Here's how the part is built. I have some questions about the finished solid (model axes, mm). A direction names the side the tool comes from. Coordinates: 2 decimals unless noted, no trailing zeros. Order: outer loops, then holes, each group sorted by start corner. A loop starts at its lowest first (then second) coordinate and runs counter-clockwise, first axis right, second up. Notation, with made-up numbers: (23.25, 82) - (77.25, 82) arc R32 ccw to (77.25, 108) - close; hole circle Ø7 at (81.25, -1). An arc over 180 degrees is marked (long way). Answer as CSV lines item,"result". Start each with the question number.
Item 1: We'd pull the mould along X, two halves only. Please class faces 4 (the face through (17.092, 32, 5)), 5 (the face through (16.52, 59.32, 1.97)), 6 (the face through (19.435, 52, 2)): pulls with the +X half, pulls with the -X half, needs draft (parallel to the pull), parting line crosses it, or undercut.
Item 2: Imagine slicing it at A-A on z = 8. List the corners of the cut face in (x, y) for me, and give its area (3 significant figures).
Item 3: Imagine slicing it at B-B on y = 33.5. List the corners of the cut face in (x, z) for me, and give its area (3 significant figures).
Item 4: Imagine slicing it at C-C on x = 21.5. List the corners of the cut face in (y, z) for me.
Item 5: I'm going to push flat-ended pins straight in: pin 1 (2 mm diameter, centred on x = 22, z = 6.5, fed in from +Y); pin 2 (5 mm diameter, centred on y = 35.5, z = 7.5, fed in from -X); pin 3 (5.5 mm diameter, centred on x = 15.44, y = 47.24, fed in from +Z). Where does each tip first touch, or does it pass through?
Item 6: Imagine slicing it at D-D on x = 19. List the corners of the cut face in (y, z) for me.
Item 7: On a 3-axis mill with a long thin cutter (end or side, diameter ignored), from which of +Z, -Z, +X, -X, +Y, -Y can I reach the whole of each face in a straight line? I mean faces 1 (the face through (22, 37.581, 7)), 2 (the face through (26.092, 32, 5)), 3 (the face through (17.4, 37.3, 6.6)). Say none if no direction works.
Item 8: I need wall thicknesses on line 1 (Y direction, x = 21.75, z = 8); line 2 (Y direction, x = 13.5, z = 2); line 3 (Y direction, x = 16.75, z = 3.75). Which ranges of each line are inside material? Lowest first, please.
Autodesk Inventor part; units mm, degrees
ref_plane "YZ Plane" through (0, 0, 0) normal (1, 0, 0) x (0, 1, 0)
ref_plane "XZ Plane" through (0, 0, 0) normal (0, 1, 0) x (-1, 0, 0)
ref_plane "XY Plane" through (0, 0, 0) normal (0, 0, 1) x (1, 0, 0)
ref_plane "Work Plane1" through (0, 0, 0) normal (0, 0, 1) x (1, 0, 0)
sketch "Sketch1" plane through (0, 0, 0) normal (0, 0, 1) x (1, 0, 0)
  circle A0 centre (-15.435, 47.2375) radius 1.95
  circle A1 centre (-15.435, 57.2375) radius 1.95
  circle A2 centre (15.435, 47.2375) radius 1.95
  circle A3 centre (15.435, 57.2375) radius 1.95
  circle A4 centre (0, -62.5) radius 13.5
  circle A5 centre (0, -43.5) radius 2
  circle A6 centre (-13.435, -49.065) radius 2
  circle A7 centre (13.435, -49.065) radius 2
  circle A8 centre (-13.435, -75.935) radius 2
  arc A9 (-14.8492, -77.3492) -> (0, -83.5) centre (0, -62.5) ccw
  circle A10 centre (0, -81.5) radius 2
  arc A11 (0, -83.5) -> (14.8492, -77.3492) centre (0, -62.5) ccw
  circle A12 centre (13.435, -75.935) radius 2
  arc A13 (14.8492, -77.3492) -> (21, -62.5) centre (0, -62.5) ccw
  circle A14 centre (19, -62.5) radius 2
  line L0 (21, 62.5) -> (21, -62.5)
  arc A15 (21, 62.5) -> (-21, 62.5) centre (0, 62.5) ccw
  line L1 (-21, -62.5) -> (-21, 62.5)
  circle A16 centre (-19, -62.5) radius 2
  arc A17 (-21, -62.5) -> (-14.8492, -77.3492) centre (0, -62.5) ccw
  circle A18 centre (-15.5, -1.9727) radius 2.1
  circle A19 centre (15.5, -1.9727) radius 2.1
  circle A20 centre (-15.5, 29.0273) radius 2.1
  circle A21 centre (15.5, 29.0273) radius 2.1
  circle A22 centre (0, 13.5273) radius 13
  line L2 (11.435, 61.2375) -> (19.435, 61.2375)
  line L3 (19.435, 61.2375) -> (19.435, 43.2375)
  line L4 (19.435, 43.2375) -> (11.435, 43.2375)
  line L5 (11.435, 43.2375) -> (11.435, 61.2375)
  circle A23 centre (15.435, 57.2375) radius 2.35
  circle A24 centre (15.435, 47.2375) radius 2.35
  line L6 (11.435, 43.2375) -> (17.0919, 37.5807)
  line L7 (11.435, 43.2375) -> (19.435, 43.2375) construction
  line L8 (19.435, 43.2375) -> (25.0919, 37.5807)
  line L9 (17.0919, 37.5807) -> (26.0919, 37.5807)
  line L10 (26.0919, 37.5807) -> (26.0919, 26.5807)
  line L11 (26.0919, 26.5807) -> (17.0919, 26.5807)
  line L12 (17.0919, 26.5807) -> (17.0919, 37.5807)
  point P0 (0, 0)
  dimension "d0" = 4
  dimension "d1" = 4
  dimension "d2" = 4
  dimension "d3" = 4
  dimension "d4" = 0.4
  dimension "d5" = 0.4
  dimension "d6" = 8
  dimension "d7" = 45
  dimension "d8" = 11
  dimension "d19" = 9
extrude "Extrusion1" add sketch "Sketch1" along normal blind 4 contours L11 L12 A21 L9 L0 | L0 L9 L10 L11 | L8 L9 L0 | L0 L9 L6 L4 L8 | L4 L5 L2 L3 | L12 A21 picked at (17.2417, 29.1915)
sketch "Sketch2" plane through (0, 0, 4) normal (0, 0, 1) x (1, 0, 0)
  line L0 (19.435, 61.2375) -> (11.435, 61.2375)
  line L1 (11.435, 61.2375) -> (11.435, 43.2375)
  line L2 (11.435, 43.2375) -> (17.0919, 37.5807)
  line L3 (17.0919, 37.5807) -> (17.0919, 26.5807)
  line L4 (17.0919, 26.5807) -> (26.0919, 26.5807)
  line L5 (26.0919, 26.5807) -> (26.0919, 37.5807)
  line L6 (25.0919, 37.5807) -> (19.435, 43.2375)
  line L7 (19.435, 43.2375) -> (19.435, 61.2375)
  circle A0 centre (15.435, 47.2375) radius 2.35
  circle A1 centre (15.435, 57.2375) radius 2.35
  line L8 (17.0919, 26.5807) -> (25.0919, 26.5807)
  line L9 (25.0919, 26.5807) -> (25.0919, 37.5807)
  line L10 (25.0919, 37.5807) -> (17.0919, 37.5807)
  line L11 (17.0919, 37.5807) -> (17.0919, 26.5807)
  line L12 (26.0919, 37.5807) -> (25.0919, 37.5807)
  point P0 (0, 0)
  point P1 (25.0919, 26.5807)
extrude "Extrusion2" add sketch "Sketch2" along normal blind 9 contours L12 L5 L4 L9 | L9 L4 L3 L10
sketch "Sketch3" plane through (26.0919, 26.5807, 0) normal (1, 0, 0) x (0, 0, -1)
  line L0 (0, 0) -> (0, 11)
  line L1 (-13, 0) -> (-13, 11)
  line L2 (0, 0) -> (-13, 0)
  circle A0 centre (-8, 5.5) radius 2.85
  line L3 (0, 11) -> (-13, 11)
  point P0 (0, -26.5807)
  dimension "d13" = 8
  dimension "d14" = 5.5
  dimension "d15" = 5.7
fillet "Fillet1" radius 2 4 edges at (11.435, 43.2375, 2) (11.435, 61.2375, 2) (19.435, 61.2375, 2) (19.435, 43.2375, 2)
extrude "Extrusion3" cut sketch "Sketch3" against normal through all contours A0
fillet "Fillet2" radius 2 2 edges at (21.5919, 37.5807, 13) (21.5919, 26.5807, 13)
fillet "Fillet3" radius 1 10 edges at (17.0919, 27.1665, 12.4142) (17.0919, 32.0807, 13) (17.0919, 36.9949, 12.4142) (17.0919, 37.5807, 7.5) (17.0919, 26.5807, 5.5) (26.0919, 27.1665, 12.4142) (26.0919, 32.0807, 13) (26.0919, 36.9949, 12.4142) (26.0919, 37.5807, 5.5) (26.0919, 26.5807, 5.5)
properties part number "top-tensioner_3DPrint"
Responses:
1,face 4,"pulls with the -X half"
1,face 5,"undercut"
1,face 6,"pulls with the +X half"
2,outline,"(17.09, 27.58) arc R1 ccw to (18.09, 26.58) - (25.09, 26.58) arc R1 ccw to (26.09, 27.58) - (26.09, 29.23) - (17.09, 29.23) - close; (17.09, 34.93) - (26.09, 34.93) - (26.09, 36.58) arc R1 ccw to (25.09, 37.58) - (18.09, 37.58) arc R1 ccw to (17.09, 36.58) - close"
2,area,"46.8 mm^2"
3,outline,"(17.09, 0) - (26.09, 0) - (26.09, 5.53) - (17.09, 5.53) - close; (17.09, 10.47) - (26.09, 10.47) - (26.09, 12) arc R1 ccw to (25.09, 13) - (18.09, 13) arc R1 ccw to (17.09, 12) - close"
3,area,"72.1 mm^2"
4,outline,"(26.58, 0) - (41.17, 0) - (41.17, 4) - (37.58, 4) - (37.58, 11) arc R2 ccw to (35.58, 13) - (28.58, 13) arc R2 ccw to (26.58, 11) - close; hole circle Ø5.7 at (32.08, 8)"
5,pin 1,"stops at y = 37.58"
5,pin 2,"stops at x = 17.09"
5,pin 3,"stops at z = 4"
6,outline,"(26.58, 0) - (60.48, 0) - (60.48, 4) - (37.58, 4) - (37.58, 11) arc R2 ccw to (35.58, 13) - (28.58, 13) arc R2 ccw to (26.58, 11) - close; hole circle Ø5.7 at (32.08, 8)"
7,face 1,"+Z, +X, -X, +Y"
7,face 2,"+Z, -Z, +X, +Y, -Y"
7,face 3,"+Z, -X"
8,line 1,"y = 26.58 to 29.23, 34.93 to 37.58"
8,line 2,"y = 41.17 to 45.9, 48.57 to 55.9, 58.57 to 61.24"
8,line 3,"y = 37.92 to 45.29, 49.19 to 55.29, 59.19 to 61.24"
